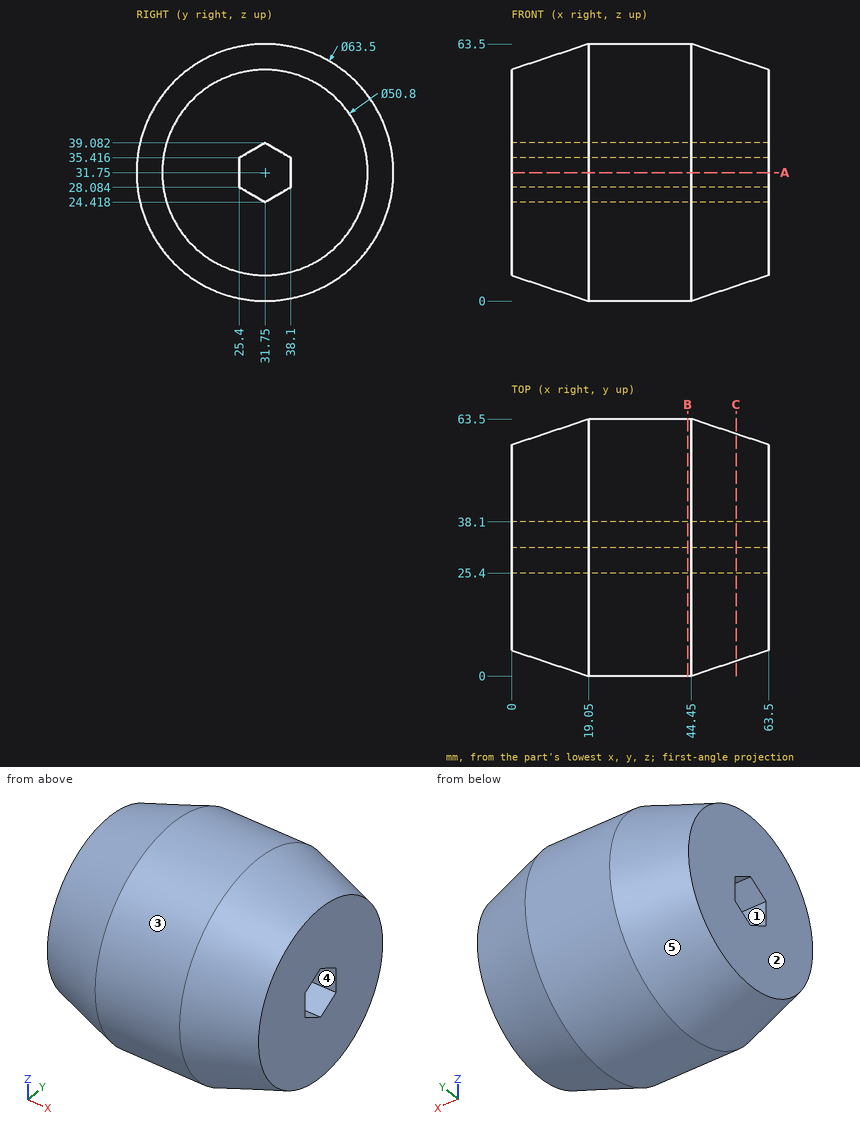
Drawing for the job (mm, zero at the part's lowest x, y, z). A direction names the side the tool comes from. Round coordinates to 2 decimals unless told otherwise and drop trailing zeros. Loops run counter-clockwise (first coordinate to the right, second up) from the corner with the lowest first, then second, coordinate; pieces in that order, holes last. Notation, with made-up numbers: (-30.5, 47.25) -> (5.5, 47.25) arc R20 ccw to (5.5, 67.25) -> close; hole circle Ø4 at (54, 33). An arc over 180 degrees is marked (long way). Answer as CSV lines item,"result". Start each with the question number.
1) Tool access for the marked faces 4 and 5: list every direction of +Z, -Z, +X, -X, +Y, -Y with a clear straight run to the whole face (end or side of a thin tool).
2) Slice it at B-B (x = 43.5). List the corners of the cut face in (y, z), plus the area to 3 significant figures.
3) Pin check, flat tips, straight feed: P1, Ø4, axis at x = 34, y = 30.5, coming from the -Z side; P2, Ø12, axis at x = 26, z = 12.5, coming from the -Y side; P3, Ø8, axis at x = 33, z = 33.5, coming from the -Y side; P4, Ø10, axis at x = 54.5, y = 9, coming from the +Z side. Stop position of each tip, or through.
4) Slice it at C-C (x = 55.5). List the corners of the cut face in (y, z).
5) Mould opens along Y. For the marked faces 1, 2 and 3 say: +Y half, -Y half, draft (parallel to the pull), parting line (faces both ways), or undercut.
6) Probe line 1 along Z through (x, y) = (55, 30.5) (1 decimal); line 2 along Y through (x, z) = (22.5, 37) (1 decimal); line 3 along Y through (x, z) = (57.5, 26.5) (1 decimal). List the from-to ranges inside material, lowest first.
7) Slice it at A-A (z = 31.75). List the corners of the cut face in (x, y), plus the area to 3 significant figures.
Filled in:
1,face 4,"+X, -X"
1,face 5,"-X"
2,outline,"circle Ø63.5 at (31.75, 31.75); hole (25.4, 28.08) -> (31.75, 24.42) -> (38.1, 28.08) -> (38.1, 35.42) -> (31.75, 39.08) -> (25.4, 35.42) -> close"
2,area,"3,030 mm2"
3,P1,"stops at z = 0"
3,P2,"stops at y = 2.9"
3,P3,"stops at y = 0"
3,P4,"stops at z = 54.45"
4,outline,"circle Ø56.13 at (31.75, 31.75); hole (25.4, 28.08) -> (31.75, 24.42) -> (38.1, 28.08) -> (38.1, 35.42) -> (31.75, 39.08) -> (25.4, 35.42) -> close"
5,face 1,"undercut"
5,face 2,"draft"
5,face 3,"parting line"
6,line 1,"z = 3.5 to 25.1, 38.4 to 60"
6,line 2,"y = 0.4 to 28.1, 35.4 to 63.1"
6,line 3,"y = 4.9 to 28.1, 35.4 to 58.6"
7,outline,"(0, 6.35) -> (19.05, 0) -> (44.45, 0) -> (63.5, 6.35) -> (63.5, 25.4) -> (0, 25.4) -> close; (0, 38.1) -> (63.5, 38.1) -> (63.5, 57.15) -> (44.45, 63.5) -> (19.05, 63.5) -> (0, 57.15) -> close"
7,area,"2,980 mm2"
